Geometry check sheet. Reference: the model listing, model coordinates, mm. A direction names the side the tool comes from. Coordinates: 2 decimals unless noted, no trailing zeros. Write each loop counter-clockwise with the first axis right and the second up, starting at its lowest first coordinate (ties: lowest second). Pieces come first, ordered by that corner, then holes. Notation, with made-up numbers: (-29.5, 46) -> (14.5, 46) arc R28 ccw to (14.5, 74) -> close; hole circle Ø10 at (12.25, 1.25). An arc over 180 degrees is marked (long way). Answer in a Markdown table with one row per item. Add a question column.
Q1. Tool access check on faces 4 (the face through (123, 5, 0)), 5 (the face through (123, 0, 4)). Record the directions out of +Z, -Z, +X, -X, +Y, -Y that give a thin tool (end or side, any length) a straight path to the whole face; none if there is none.
Q2. Gauge pin test, flat end, axial feed: P1, Ø1.8, axis at x = 235, z = 0, coming from the -Y side. Record the tip position at first contact, or that the pin passes through.
Q3. Thickness scan on line 1 (X direction, y = 4.75, z = -0.25); line 2 (Z direction, x = 44, y = 2.25); line 3 (Y direction, x = 39, z = -4.3). Record the ranges inside material, lowest first.
Q4. Release check for a two-part mould opening along Z. For faces 1 (the face through (123, -5, 0)), 2 (the face through (123, 0, -5)), 3 (the face through (123, 4, 0)) record: pulls with the +Z half, pulls with the -Z half, needs draft (parallel to the pull), parting line crosses it, or undercut.
Q5. Section check C-C, the plane y = 0. Count the separate pieces of the cut face and the enclosed holes in it, and give its area (3 significant figures).
Q6. Section check A-A, the plane z = 0. Record the boundary of the cut face in (x, y), and give its area (3 significant figures).
Q7. Section check B-B, the plane x = 231. Record the boundary of the cut face in (y, z), and give its area (3 significant figures).
Autodesk Inventor part; units mm, degrees
ref_plane "YZ Plane" through (0, 0, 0) normal (1, 0, 0) x (0, 1, 0)
ref_plane "XZ Plane" through (0, 0, 0) normal (0, 1, 0) x (-1, 0, 0)
ref_plane "XY Plane" through (0, 0, 0) normal (0, 0, 1) x (1, 0, 0)
sketch "スケッチ1" plane through (0, 0, 0) normal (1, 0, 0) x (0, 1, 0)
  line L0 (5, 5) -> (-5, 5)
  line L1 (-5, 5) -> (-5, -5)
  line L2 (-5, -5) -> (5, -5)
  line L3 (5, -5) -> (5, 5)
  line L4 (4, 4) -> (-4, 4)
  line L5 (-4, 4) -> (-4, -4)
  line L6 (-4, -4) -> (4, -4)
  line L7 (4, -4) -> (4, 4)
  point P0 (0, 0)
  dimension "d0" = 1
  dimension "d1" = 1
  dimension "d2" = 1
  dimension "d3" = 1
  dimension "d4" = 10
  dimension "d5" = 10
  dimension "d6" = 5
  dimension "d7" = 5
extrude "押し出し1" add sketch "スケッチ1" along normal blind 250
sketch "スケッチ2" plane through (0, -5, 5) normal (0, 0, 1) x (1, 0, 0)
  circle A0 centre (60, 5) radius 1.5
  circle A1 centre (190, 5) radius 1.5
  line L0 (250, 10) -> (250, 0)
  line L1 (0, 10) -> (0, 0)
  line L2 (0, 0) -> (250, 0)
  point P0 (0, 5)
  dimension "d10" = 60
  dimension "d11" = 3
  dimension "d12" = 3
  dimension "d13" = 60
  dimension "d14" = 5
extrude "押し出し2" cut sketch "スケッチ2" against normal blind 200
sketch "スケッチ3" plane through (0, -5, 5) normal (0, 0, 1) x (1, 0, 0)
  circle A0 centre (5, 5) radius 1.5
  circle A1 centre (245, 5) radius 1.5
  line L0 (250, 10) -> (250, 0)
  line L1 (0, 10) -> (250, 10)
  line L2 (0, 10) -> (0, 0)
  point P0 (0, 5)
  dimension "d17" = 5
  dimension "d18" = 5
  dimension "d19" = 3
  dimension "d20" = 5
  dimension "d21" = 5
  dimension "d22" = 3
extrude "押し出し3" cut sketch "スケッチ3" against normal blind 200
sketch "スケッチ4" plane through (0, -5, 5) normal (0, 0, 1) x (1, 0, 0)
  circle A0 centre (39, 5) radius 1.5
  circle A1 centre (60, 5) radius 1.5
  circle A2 centre (211, 5) radius 1.5
  circle A3 centre (190, 5) radius 1.5
  point P0 (0, 5)
  dimension "d25" = 3
  dimension "d26" = 21
  dimension "d27" = 3
  dimension "d28" = 21
extrude "押し出し4" cut sketch "スケッチ4" against normal blind 200 contours A0 | A2
sketch "スケッチ5" plane through (0, 5, 5) normal (0, 1, 0) x (1, 0, 0)
  circle A0 centre (15, 5) radius 1.5
  line L0 (0, 10) -> (250, 10)
  line L1 (0, 10) -> (0, 0)
  circle A1 centre (235, 5) radius 1.5
  line L2 (250, 10) -> (250, 0)
  line L3 (0, 0) -> (250, 0)
  point P0 (0, 5)
  dimension "d31" = 3
  dimension "d32" = 5
  dimension "d33" = 15
  dimension "d34" = 15
  dimension "d35" = 5
  dimension "d36" = 3
extrude "押し出し5" cut sketch "スケッチ5" against normal blind 200 contours A0 | A1
properties part number "f&bparts" material "アルミニウム 6061"
Calculated:
| question | item | result |
|---|---|---|
| 1 | face 4 | +Z, -Z, +X, -X, +Y |
| 1 | face 5 | +X, -X |
| 2 | P1 | passes through |
| 3 | line 1 | x = 0 to 13.52, 16.48 to 233.52, 236.48 to 250 |
| 3 | line 2 | z = -5 to -4, 4 to 5 |
| 3 | line 3 | y = -5 to -1.5, 1.5 to 5 |
| 4 | face 1 | needs draft |
| 4 | face 2 | pulls with the -Z half |
| 4 | face 3 | undercut |
| 5 | separate pieces | 14 |
| 5 | enclosed holes | 0 |
| 5 | area | 464 mm² |
| 6 | outline | (0, -5) -> (13.5, -5) -> (13.5, -4) -> (0, -4) -> close; (0, 4) -> (13.5, 4) -> (13.5, 5) -> (0, 5) -> close; (16.5, -5) -> (233.5, -5) -> (233.5, -4) -> (16.5, -4) -> close; (16.5, 4) -> (233.5, 4) -> (233.5, 5) -> (16.5, 5) -> close; (236.5, -5) -> (250, -5) -> (250, -4) -> (236.5, -4) -> close; (236.5, 4) -> (250, 4) -> (250, 5) -> (236.5, 5) -> close |
| 6 | area | 488 mm² |
| 7 | outline | (-5, -5) -> (5, -5) -> (5, 5) -> (-5, 5) -> close; hole (-4, -4) -> (4, -4) -> (4, 4) -> (-4, 4) -> close |
| 7 | area | 36.0 mm² |
